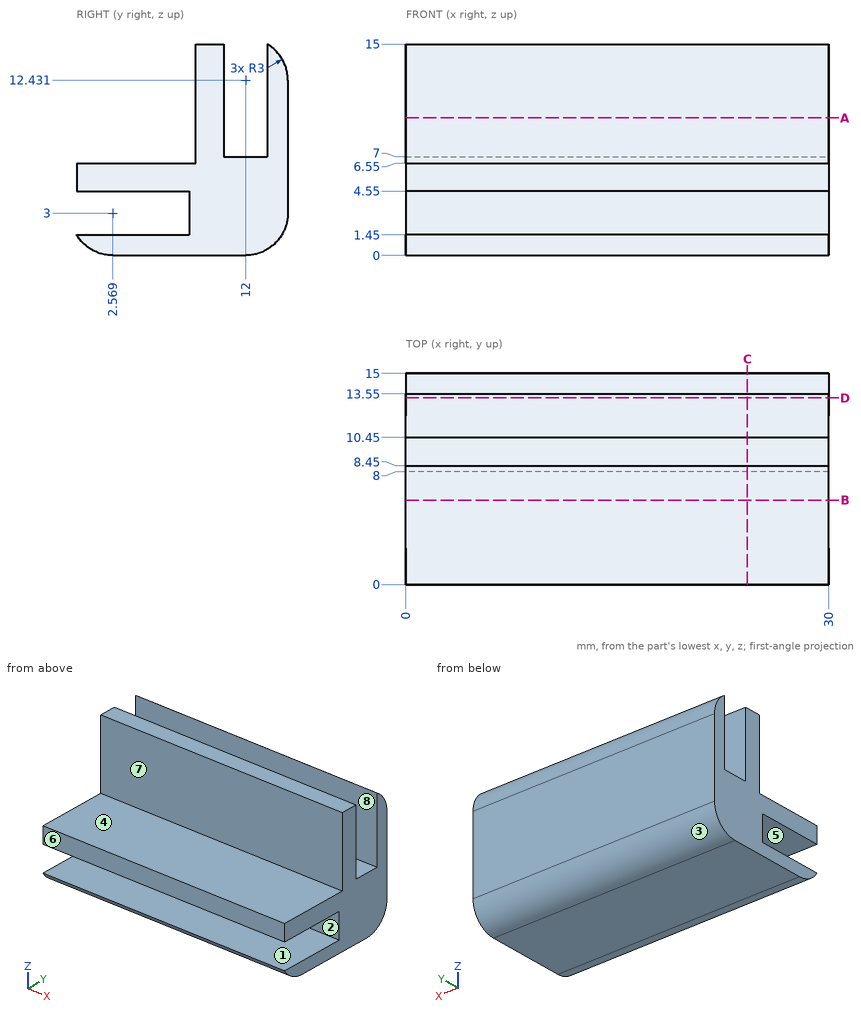
Print and shaded views of the part. All mm, measured from the part's lowest x, y and z. A direction names the side the tool comes from. Give positions to 0.01 mm unless a question says otherwise; leave off trailing zeros. Write each loop counter-clockwise with the first axis right and the second up, starting at its lowest first coordinate (ties: lowest second). Pieces come first, ordered by that corner, then holes. Notation, with made-up numbers: (-26, -22.75) -> (8, -22.75) arc R21 cw to (8, -13.75) -> close; hole circle Ø7 at (71.25, 51). An arc over 180 degrees is marked (long way). Use CSV: the item, a comma, the result in double quotes. Start each with the question number.
1) Pin check, flat tips, straight feed: P1, Ø3, axis at x = 25.5, y = 2, coming from the -Z side; P2, Ø2.5, axis at x = 21.5, z = 3, coming from the -Y side; P3, Ø2.5, axis at x = 8.5, y = 2.5, coming from the +Z side; P4, Ø2.5, axis at x = 10.5, z = 10.5, coming from the -Y side. Stop position of each tip, or through.
2) Cut at B-B on y = 6. List the corners of the cut face in (x, z).
3) Drill centre lines: L1, parallel to Y at x = 5.5, z = 7.5; L2, parallel to Z at x = 25, y = 5.5; L3, parallel to Y at x = 8.75, z = 14. Where is each one in solid material? Low to high.
4) Tool access for the marked faces 5, 6, 7 and 8: list every direction of +Z, -Z, +X, -X, +Y, -Y with a clear straight run to the whole face (end or side of a thin tool).
5) Two-plate mould, pull along Z, no slides. Class the marked faces 1, 2, 3 and 4: released by +Z, released by -Z, zero draft, split by the parting line, or undercut.
6) Cut at A-A on z = 9.75. List the corners of the cut face in (x, y).
7) Cut at D-D on y = 13.25. List the corners of the cut face in (x, z).
8) Cut at C-C on x = 24.25. List the corners of the cut face in (y, z).
Final values:
1,P1,"stops at z = 0"
1,P2,"stops at y = 8"
1,P3,"stops at z = 6.55"
1,P4,"stops at y = 8.45"
2,outline,"(0, 0) -> (30, 0) -> (30, 1.45) -> (0, 1.45) -> close; (0, 4.55) -> (30, 4.55) -> (30, 6.55) -> (0, 6.55) -> close"
3,L1,"y = 8.45 to 10.45, 13.55 to 15"
3,L2,"z = 0 to 1.45, 4.55 to 6.55"
3,L3,"y = 8.45 to 10.45, 13.55 to 14.56"
4,face 5,"+X, -X, -Y"
4,face 6,"+Z, -Z, +X, -X, -Y"
4,face 7,"+Z, +X, -X, -Y"
4,face 8,"+Z, +X, -X"
5,face 1,"undercut"
5,face 2,"undercut"
5,face 3,"released by -Z"
5,face 4,"released by +Z"
6,outline,"(0, 8.45) -> (30, 8.45) -> (30, 10.45) -> (0, 10.45) -> close; (0, 13.55) -> (30, 13.55) -> (30, 15) -> (0, 15) -> close"
7,outline,"(0, 0.27) -> (30, 0.27) -> (30, 7) -> (0, 7) -> close"
8,outline,"(0, 1.45) arc R3 ccw to (2.57, 0) -> (12, 0) arc R3 ccw to (15, 3) -> (15, 12.43) arc R3 ccw to (13.55, 15) -> (13.55, 7) -> (10.45, 7) -> (10.45, 15) -> (8.45, 15) -> (8.45, 6.55) -> (0, 6.55) -> (0, 4.55) -> (8, 4.55) -> (8, 1.45) -> close"
